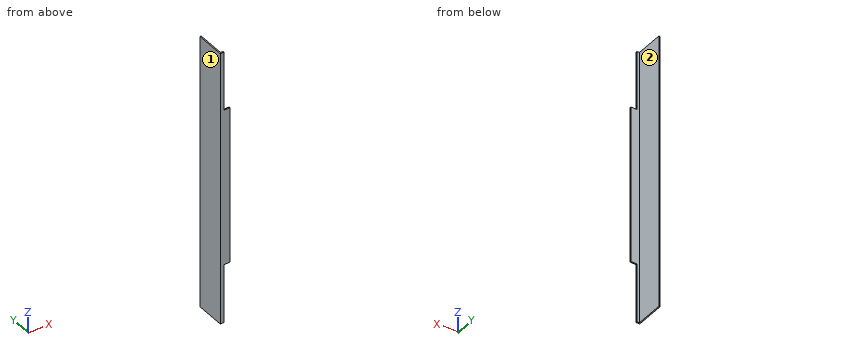
Autodesk Inventor part; units mm, degrees
ref_plane "YZ Plane" through (0, 0, 0) normal (1, 0, 0) x (0, 1, 0)
ref_plane "XZ Plane" through (0, 0, 0) normal (0, 1, 0) x (-1, 0, 0)
ref_plane "XY Plane" through (0, 0, 0) normal (0, 0, 1) x (1, 0, 0)
sketch "Sketch1" plane through (0, 0, 0) normal (0, 0, 1) x (1, 0, 0)
  line L0 (0, 0) -> (25.4, 0)
  line L1 (25.4, 0) -> (25.4, 3.175)
  line L2 (3.175, 76.2) -> (0, 76.2)
  line L3 (0, 76.2) -> (0, 0)
  line L4 (3.175, 76.2) -> (3.175, 3.175)
  line L5 (3.175, 3.175) -> (25.4, 3.175)
  dimension "d0" = 76.2
  dimension "d1" = 25.4
  dimension "d2" = 3.175
  dimension "d3" = 3.175
extrude "Extrusion1" add sketch "Sketch1" along normal blind 711.2
sketch "Sketch2" plane through (0, 0, 0) normal (0, -1, 0) x (1, 0, 0)
  line L0 (0, 0) -> (0, 711.2)
  line L1 (25.4, 0) -> (25.4, 711.2)
  line L2 (0, 355.6) -> (25.4, 355.6)
  line L3 (25.4, 0) -> (9.525, 0)
  line L4 (9.525, 0) -> (9.525, 152.4)
  line L5 (9.525, 152.4) -> (25.4, 152.4)
  line L6 (25.4, 152.4) -> (25.4, 0)
  line L7 (25.4, 711.2) -> (9.525, 711.2)
  line L8 (9.525, 711.2) -> (9.525, 558.8)
  line L9 (9.525, 558.8) -> (25.4, 558.8)
  line L10 (25.4, 558.8) -> (25.4, 711.2)
  dimension "d7" = 15.875
  dimension "d8" = 152.4
extrude "Extrusion2" cut sketch "Sketch2" against normal through all
equation "\"d3\" = d2"
properties part number "frame 7 outside L"
Input: part model. Units: mm. Frame: model coordinates. Face numbers are marked on the shaded views. A direction names the side the tool comes from. Coordinates: 2 decimals unless noted, no trailing zeros. Loops run counter-clockwise (first coordinate to the right, second up) from the corner with the lowest first, then second, coordinate; pieces in that order, holes last. Notation, with made-up numbers: (77.25, 37) -> (92.25, 37) arc R23 ccw to (92.25, 55) -> close; hole circle Ø11 at (-8.5, 15). An arc over 180 degrees is marked (long way). One line per item, written item: value.
(1) Cut plane A-A (z = 320). Output: boundary loops of the cut face in (x, y) (3 decimals).
Answer below:
outline: (0, 0) -> (25.4, 0) -> (25.4, 3.175) -> (3.175, 3.175) -> (3.175, 76.2) -> (0, 76.2) -> close
(2) Ray query, line 1 along X through (y, z) = (34.5, 419.5) (3 decimals). Return the intervals inside material, ascending.
Answer below:
line 1: x = 0 to 3.175
(3) Pin query (flat end, axial travel): pin 1 Ø1 at (y, z) = (1.5, 597.5) entering from +X (3 decimals); pin 2 Ø1 at (x, y) = (13.5, 2) entering from +Z; pin 3 Ø8 at (x, y) = (3.5, 67) entering from +Z; pin 4 Ø22 at (y, z) = (47.5, 276.5) entering from +X (3 decimals). Return the tip coordinate at first contact, or that it passes through.
Answer below:
pin 1: stops at x = 9.525
pin 2: stops at z = 558.8
pin 3: stops at z = 711.2
pin 4: stops at x = 3.175
(4) Cut plane B-B (x = 20). Output: boundary loops of the cut face in (y, z) (3 decimals), then the cut area to 3 significant figures.
Answer below:
outline: (0, 152.4) -> (3.175, 152.4) -> (3.175, 558.8) -> (0, 558.8) -> close
area: 1,290 mm2
(5) Cut plane D-D (z = 89). Output: boundary loops of the cut face in (x, y) (3 decimals), then the cut area to 3 significant figures.
Answer below:
outline: (0, 0) -> (9.525, 0) -> (9.525, 3.175) -> (3.175, 3.175) -> (3.175, 76.2) -> (0, 76.2) -> close
area: 262 mm2
(6) Cut plane C-C (y = 19). Output: boundary loops of the cut face in (x, z) (3 decimals).
Answer below:
outline: (0, 0) -> (3.175, 0) -> (3.175, 711.2) -> (0, 711.2) -> close
(7) Set-up query: the marked faces 1 and 2. Return all of +Z, -Z, +X, -X, +Y, -Y with unobstructed straight access to the full face (end or side cutting, diameter ignored); none if empty.
Answer below:
face 1: +Z, -Z, -X, +Y, -Y
face 2: +Z, -Z, +X, +Y
